```python
from build123d import *

# Parameters (mm, degrees)
SKETCH1_W               = 8
SKETCH1_H               = 8
BOSS_EXTRUDE1_DEPTH     = 3
CUT_EXTRUDE1_DEPTH      = 12.704699911
CUT_EXTRUDE1_DEPTH_BACK = 12.704699911
CUT_EXTRUDE2_DEPTH      = 11
SKETCH4_R               = 1.8
CUT_EXTRUDE3_DEPTH      = 0.8
SKETCH5_W               = 8
SKETCH5_H               = 1
BOSS_EXTRUDE2_DEPTH     = 2
FILLET1_R               = 4
CUT_EXTRUDE4_DEPTH      = 0.4


with BuildPart() as part:
    # Sketch1 → Boss-Extrude1 (new body)
    with BuildSketch(Plane(origin=(0, 0, 0), x_dir=(1, 0, 0), z_dir=(0, 1, 0))):
        with Locations((4, 4)):
            Rectangle(SKETCH1_W, SKETCH1_H)
    extrude(amount=BOSS_EXTRUDE1_DEPTH)

    # Sketch2 → Cut-Extrude1 (cut, two sides: drawn at the far end of the back side and taken through both)
    with BuildSketch(Plane.XY.offset(-CUT_EXTRUDE1_DEPTH_BACK)):
        Polygon((0, 0), (0.6, 3), (0, 3), align=None)
        Polygon((8, 0), (7.4, 3), (8, 3), align=None)
    extrude(amount=CUT_EXTRUDE1_DEPTH + CUT_EXTRUDE1_DEPTH_BACK, mode=Mode.SUBTRACT)

    # Sketch3 → Cut-Extrude2 (cut)
    with BuildSketch(Plane(origin=(0, 0, 0), x_dir=(0, 0, -1), z_dir=(1, 0, 0))):
        Polygon((0, 0), (0.6, 3), (0, 3), align=None)
        Polygon((8, 3), (7.4, 3), (8, 0), align=None)
    extrude(amount=CUT_EXTRUDE2_DEPTH, mode=Mode.SUBTRACT)

    # Sketch4 → Cut-Extrude3 (cut)
    with BuildSketch(Plane.XZ):
        with Locations(Location((4, -3.75, 0), (0, 0, 270))):
            Circle(SKETCH4_R)
    extrude(amount=-CUT_EXTRUDE3_DEPTH, mode=Mode.SUBTRACT)

    # Sketch5 → Boss-Extrude2 (add)
    with BuildSketch(Plane.XZ):
        with Locations((4, -7.5)):
            Rectangle(SKETCH5_W, SKETCH5_H)
    extrude(amount=BOSS_EXTRUDE2_DEPTH)

    # Fillet1
    # the kernel refuses this fillet: 4 mm, written as the material it takes off along each edge
    with BuildSketch(Plane(origin=(8, -2, -16.660254038), x_dir=(0, 1, 0), z_dir=(0, 0, 1)), Plane(origin=(0, -2, 1.660254038), x_dir=(0, 1, 0), z_dir=(0, 0, -1))) as fillet1_piece_1:
        with BuildLine():
            CenterArc((4, 3.464101615), FILLET1_R, 180, 60)
            Line((0, 3.464101615), (-0.08, 3.464101615))
            Line((-0.08, 3.464101615), (-0.08, 0))
            Line((-0.08, 0), (0, -0.08))
            ThreePointArc((0, -0.08), (1, -0.08), (1.96, -0.069282032))
            Line((1.96, -0.069282032), (2, 0))
        make_face()
    extrude(amount=18.320508076, mode=Mode.SUBTRACT)

    # Sketch6 → Cut-Extrude4 (cut)
    with BuildSketch(Plane(origin=(0, 3, 0), x_dir=(1, 0, 0), z_dir=(0, 1, 0))):
        Polygon((2.459405501, 2.064543337), (2.459405501, 6.064543337), (3.22863627, 6.064543337), (3.22863627, 4.474799747), (4.869661911, 4.474799747), (4.869661911, 6.064543337), (5.63889268, 6.064543337), (5.63889268, 2.064543337), (4.869661911, 2.064543337), (4.869661911, 3.80813308), (3.22863627, 3.80813308), (3.22863627, 2.064543337), align=None)
    extrude(amount=-CUT_EXTRUDE4_DEPTH, mode=Mode.SUBTRACT)


solid = part.part
```
The listing builds one solid part. Answer for the finished solid, in the listing's coordinates (mm). A direction names the side the tool comes from. Give positions to 0.01 mm unless a question says otherwise; leave off trailing zeros. Order: outer loops, then holes, each group sorted by start corner. A loop starts at its lowest first (then second) coordinate and runs counter-clockwise, first axis right, second up. Notation, with made-up numbers: (24, 69.25) -> (30, 69.25) arc R26 ccw to (30, 95.25) -> close; hole circle Ø6 at (-13.75, 75). An arc over 180 degrees is marked (long way). Answer as a JSON object with one key per item and string values. Group by question number.
Item 1: Determine the mould class of faces 4 (the cylindrical face through (4.541, 0.394, -5.467)), 5 (the flat face through (3, 0, -2)), 6 (the flat face through (4, -1, -8)) for opening direction Z: pulls with the +Z half, pulls with the -Z half, needs draft (parallel to the pull), parting line crosses it, or undercut.
Item 2: Flat-ended cylindrical pins translate along their axes: pin 1 (1 mm diameter, centred on x = 5.5, y = -1.5, fed in from +Z); pin 2 (4.5 mm diameter, centred on x = 4, z = -3.75, fed in from -Y). Find the tip coordinate at first contact, or state that the pin passes through.
Item 3: The part is cut by section A-A on x = 4. Write down the section's boundary in (y, z), and give its area (3 significant figures).
Item 4: The part is cut by section B-B on z = -3.25. Write down the section's boundary in (x, y).
Item 5: The part is cut by section D-D on x = 5.5. Write down the section's boundary in (y, z).
Item 6: A tool of negligible diameter and unlimited length cuts with its end or side. For faces 1 (the flat face through (4, 0.8, -4)), 2 (the flat face through (4, 3, -5)), 3 (the flat face through (4, -1, -7)), from which of +Z, -Z, +X, -X, +Y, -Y can it reach the whole face along a straight path? Write none if from no direction.
Item 7: The part is cut by section C-C on y = 2.1. Write down the section's boundary in (x, z), and give its area (3 significant figures).
Item 8: Consider L1, parallel to Y at x = 5.25, z = -4.5; L2, parallel to Y at x = 1, z = -4.75; L3, parallel to X at y = 0.4, z = -3.75. Determine where each line is inside the solid, lowest interval first. Write a range as from..to.
Result set:
{
 "1": {"face 4": "undercut", "face 5": "needs draft", "face 6": "pulls with the -Z half"},
 "2": {"pin 1": "z = -7", "pin 2": "y = 0"},
 "3": {"outline": "(-2, -8) -> (0, -8) -> (3, -7.4) -> (3, -4.47) -> (2.6, -4.47) -> (2.6, -3.81) -> (3, -3.81) -> (3, -0.6) -> (0, 0) -> (0, -1.95) -> (0.8, -1.95) -> (0.8, -5.55) -> (0, -5.55) -> (0, -7) -> (-2, -7) -> close", "area": "21.1 mm²"},
 "4": {"outline": "(0, 0) -> (2.27, 0) -> (2.27, 0.8) -> (5.73, 0.8) -> (5.73, 0) -> (8, 0) -> (7.4, 3) -> (5.64, 3) -> (5.64, 2.6) -> (4.87, 2.6) -> (4.87, 3) -> (3.23, 3) -> (3.23, 2.6) -> (2.46, 2.6) -> (2.46, 3) -> (0.6, 3) -> close"},
 "5": {"outline": "(-1.88, -8) -> (0, -8) -> (3, -7.4) -> (3, -6.06) -> (2.6, -6.06) -> (2.6, -2.06) -> (3, -2.06) -> (3, -0.6) -> (0, 0) -> (0, -2.76) -> (0.8, -2.76) -> (0.8, -4.74) -> (0, -4.74) -> (0, -7) -> (-1.88, -7) -> close"},
 "6": {"face 1": "-Y", "face 2": "+Z, -Z, +X, -X, +Y", "face 3": "+Z, +X, -X, -Y"},
 "7": {"outline": "(0.42, -7.58) -> (7.58, -7.58) -> (7.58, -0.42) -> (0.42, -0.42) -> close", "area": "51.3 mm²"},
 "8": {"L1": "0.8..2.6", "L2": "0..3", "L3": "0.08..2.2, 5.8..7.92"}
}
